The listing builds one solid part. Answer for the finished solid, in the listing's coordinates (mm). A direction names the side the tool comes from. Round coordinates to 2 decimals unless told otherwise and drop trailing zeros. Write each loop counter-clockwise with the first axis right and the second up, starting at its lowest first coordinate (ties: lowest second). Pieces come first, ordered by that corner, then holes. Notation, with made-up numbers: M -5.75,-21 L 0.25,-21 A26 cw 0.25,13 Z; hole C -31.75,13.25 d1. An arc over 180 degrees is marked long. One line per item, written item: value. Start each with the question number.
(1) Section A-A (y = -38.1) is taken. Determine the outline of the cut face in (x, z), plus the area to 3 significant figures.
(2) Section B-B (x = -29.5) is taken. Determine the outline of the cut face in (y, z).
(3) For faces 4 (the flat face through (-31, -32, -158.134)), 5 (the flat face through (-31, -31, -132.734)), 6 (the flat face through (-12.7, -38, -145)), determine the directions among +Z, -Z, +X, -X, +Y, -Y from which every point of the face is accessible in a straight line to the end or side of a thin tool.
(4) For a pull along Y with two mould halves and no side action, classify faces 1 (the conical face through (-6.4, -102.4, -127)), 2 (the flat face through (-102, 12.7, -133)), 3 (the flat face through (0, -75, -135)) as released by +Y, released by -Y, zero draft, split by the parting line, or undercut.
(5) Consider probe 1 along Z at (x, y) = (-17.5, -67); probe 2 along Y at (x, z) = (-40, -153); probe 3 along Y at (x, z) = (-63, -147). Determine where each line is inside the solid, lowest interval first.
(6) Given P1, Ø10, axis at x = -33, y = -50.5, coming from the +Z side; P2, Ø11.5, axis at y = -101.5, z = -131, coming from the +X side; P3, Ø12, axis at y = -64.5, z = -118, coming from the -X side; P4, Ø4, axis at y = -120, z = -106.5, coming from the -X side, each flat-ended and moving along its own axis, determine where each tip first touches the part or whether it passes through.
(7) Section C-C (x = -88) is taken. Determine the outline of the cut face in (y, z), plus the area to 3 significant figures.
(8) Section D-D (y = -3.5) is taken. Determine the outline of the cut face in (x, z), plus the area to 3 significant figures.
```python
from build123d import *

# Parameters (mm, degrees)
F1_ANGLE = 90
F3_R     = 6.35
F4_DEPTH = 12.7
F4_TAPER = 5
F5_R     = 6.35
F6_DEPTH = 12.7
F6_TAPER = 5


# Not quite as in the source:
# - a feature of the source that left no trace in its solid (it failed there, or was rolled back) is left out


with BuildPart() as f1:
    # F0 (on Front) → F1 (revolve)
    with BuildSketch(Plane.XZ):
        with BuildLine():
            Line((-81.28, -158.1341253493), (0, -158.1341253493))
            Line((0, -158.1341253493), (0, -132.7341253493))
            Line((0, -132.7341253493), (-77.331499878, -132.7341253493))
            ThreePointArc((-77.331499878, -132.7341253493), (-94.9330399433, -120.7734525165), (-110.7127485092, -106.4950525761))
            Line((-110.7127485092, -106.4950525761), (-125.4562139511, -106.4950525761))
            Line((-125.4562139511, -106.4950525761), (-125.5056119373, -106.4950525761))
            ThreePointArc((-125.5056119373, -106.4950525761), (-128.3196475153, -103.0869677141), (-131.041165147, -99.6045575657))
            Line((-131.041165147, -99.6045575657), (-147.2812687077, -99.6045575657))
            ThreePointArc((-147.2812687077, -99.6045575657), (-117.9681777623, -133.0276250839), (-81.28, -158.1341253493))
        make_face()
    revolve(axis=Axis((0, 0, -145.4341253493), (0, 0, 1)), revolution_arc=F1_ANGLE)

    # F3 (on face) → F4 (join)
    with BuildSketch(Plane.XZ):
        with Locations((-101.6, -132.7341253493)):
            Circle(F3_R)
        with Locations((-38.1, -145.4341253493)):
            Circle(F3_R)
    extrude(amount=-F4_DEPTH, taper=F4_TAPER)

    # F5 (on face) → F6 (cut)
    with BuildSketch(Plane.YZ):
        with Locations((-101.6, -132.7341253493)):
            Circle(F5_R)
        with Locations((-38.1, -145.4341253493)):
            Circle(F5_R)
    extrude(amount=-F6_DEPTH, taper=F6_TAPER, mode=Mode.SUBTRACT)


solid = f1.part
```
Recorded:
1. outline: M -142.27,-99.6 A173.67 ccw -71.8,-158.13 L 0,-158.13 L 0,-151.78 L -12.7,-150.67 L -12.7,-140.2 L 0,-139.08 L 0,-132.73 L -67.29,-132.73 A148.82 cw -103.95,-106.5 L -119.58,-106.5 A160.13 cw -125.38,-99.6 Z
1. area: 3,350 mm2
2. outline: M -144.3,-99.6 A175.34 ccw -75.74,-158.13 L 0,-158.13 L 0,-132.73 L -71.48,-132.73 A150.76 cw -106.71,-106.5 L -121.99,-106.5 A161.93 cw -127.68,-99.6 Z
3. face 4: -Z, +X, -X, +Y, -Y
3. face 5: +Z, +X, +Y
3. face 6: +X
4. face 1: undercut
4. face 2: released by +Y
4. face 3: zero draft
5. probe 1: z = -158.13 to -132.73
5. probe 2: y = -81.26 to 0
5. probe 3: y = -77.68 to 0
6. P1: stops at z = -132.73
6. P2: stops at x = 0
6. P3: stops at x = -122.91
6. P4: stops at x = -80.67
7. outline: M -118.1,-99.6 A154.5 ccw 0,-154.5 L 0,-125.91 A125.91 cw -67.18,-106.5 L -89.49,-106.5 A139.1 cw -97.1,-99.6 Z
7. area: 2,980 mm2
8. outline: M -147.24,-99.6 A177.77 ccw -81.2,-158.13 L 0,-158.13 L 0,-132.73 L -77.25,-132.73 A153.58 cw -110.66,-106.5 L -125.46,-106.5 A164.56 cw -130.99,-99.6 Z
8. area: 3,620 mm2
